Source: CAD feature listing. Evaluate the final solid. Frame: model axes, mm. A direction names the side the tool comes from. Give positions to 0.01 mm unless a question says otherwise; leave off trailing zeros. Write each loop counter-clockwise with the first axis right and the second up, starting at its lowest first coordinate (ties: lowest second). Pieces come first, ordered by that corner, then holes. Notation, with made-up numbers: (19.25, 14) -> (55.25, 14) arc R31 cw to (55.25, 46) -> close; hole circle Ø1 at (76.25, 79.5). An arc over 180 degrees is marked (long way). Answer as a JSON object with one key per item and string values. Group by question number.
Item 1: First-contact query: pin 1 Ø5 at (x, z) = (40.5, -44.5) entering from +Y; pin 2 Ø1.7 at (y, z) = (15, -40.9) entering from +X; pin 3 Ø4 at (y, z) = (14, -47) entering from -X; pin 4 Ø4 at (x, y) = (29.5, 23) entering from -Z. Flat tips, straight axial feed; report the tip coordinate or a pass-through.
Item 2: Access query for faces 4 (the face through (43.5, 17.7, -54.8)), 5 (the face through (45.2, 15, -41)), 6 (the face through (32, 15, -6)), 7 (the face through (19.8, 22, -43)). Directions: +Z, -Z, +X, -X, +Y, -Y. A direction counts if a zero-diameter tool reaches every point of the face in a straight line with its end or side. Return the directions, or none.
Item 3: Section query A-A on z = -48.34. Return the cut outline in (x, y), plus the area to 3 significant figures.
Item 4: Section query B-B on y = 15. Return the cut outline in (x, z), plus the area to 3 significant figures.
Item 5: Section query D-D on y = 5.5. Return the cut outline in (x, z), plus the area to 4 significant figures.
Item 6: Section query C-C on z = -30. Return the cut outline in (x, y), plus the area to 3 significant figures.
Item 7: Ray query, probe 1 along X at (y, z) = (25, -13); probe 2 along Y at (x, z) = (43.25, -48.34); probe 3 along Y at (x, z) = (47.75, -40.9). Return the intervals inside material, ascending. Write a range as from..to.
Item 8: Pull-direction query (Z, two-part tool) for faces 1 (the face through (31, 15, -11)), 2 (the face through (41.6, 22, -43)), 3 (the face through (47.228, 15.279, -56.667)); classes: pulls with the +Z half, pulls with the -Z half, needs draft (parallel to the pull), parting line crosses it, or undercut.
from build123d import *

# Parameters (mm, degrees)
SKETCH1_W           = 5
SKETCH1_H           = 70
SKETCH1_W_2         = 40
SKETCH1_H_2         = 5
BOSS_EXTRUDE1_DEPTH = 30
SKETCH2_R           = 7
CUT_EXTRUDE1_DEPTH  = 70
SKETCH3_W           = 111.167782235
SKETCH3_H           = 40.74685258
CUT_EXTRUDE2_DEPTH  = 0.8
SKETCH5_W           = 117.774687649
SKETCH5_H           = 158.291815666
CUT_EXTRUDE3_DEPTH  = 0.8
SKETCH6_W           = 70
SKETCH6_H           = 30
BOSS_EXTRUDE2_DEPTH = 3.4
SKETCH7_W           = 70
SKETCH7_H           = 30
BOSS_EXTRUDE3_DEPTH = 6.7
SKETCH8_W           = 83.763231722
SKETCH8_H           = 77.916949986
CUT_EXTRUDE5_DEPTH  = 6
SKETCH9_R           = 7
CUT_EXTRUDE6_DEPTH  = 90.354574589
SKETCH10_W          = 29.9
SKETCH10_H          = 30
BOSS_EXTRUDE4_DEPTH = 6
SKETCH11_W          = 55.967068903
SKETCH11_H          = 62.229878259
CUT_EXTRUDE7_DEPTH  = 6
SKETCH12_W          = 64
SKETCH12_H          = 30
BOSS_EXTRUDE6_DEPTH = 4.05
SKETCH13_W          = 85.617860434
SKETCH13_H          = 123.38327663
CUT_EXTRUDE9_DEPTH  = 4.05
SKETCH15_W          = 39.049263631
SKETCH15_H          = 151.632152685
CUT_EXTRUDE10_DEPTH = 3.95
SKETCH16_W          = 64
SKETCH16_H          = 30
BOSS_EXTRUDE7_DEPTH = 4.05
SKETCH17_W          = 96.474130843
SKETCH17_H          = 104.566259817
CUT_EXTRUDE11_DEPTH = 4.05
SKETCH18_W          = 6.755230809
SKETCH18_H          = 55.059186595
CUT_EXTRUDE12_DEPTH = 4.05
SKETCH19_R          = 7
CUT_EXTRUDE14_DEPTH = 34.05
SKETCH23_W          = 19.849593964
SKETCH23_H          = 19.85515092
BOSS_EXTRUDE9_DEPTH = 4.2
SKETCH24_R          = 0.93
CUT_EXTRUDE16_DEPTH = 4
SKETCH24_5_R        = 0.93
CUT_EXTRUDE17_DEPTH = 4
SKETCH26_R          = 7
CUT_EXTRUDE18_DEPTH = 0.4


with BuildPart() as part:
    # Sketch1 → Boss-Extrude1 (new body)
    with BuildSketch(Plane(origin=(0, 0, 0), x_dir=(1, 0, 0), z_dir=(0, 1, 0))):
        with Locations((2.5, 40)):
            Rectangle(SKETCH1_W, SKETCH1_H)
        with Locations((25, 2.5)):
            Rectangle(SKETCH1_W_2, SKETCH1_H_2)
        with Locations((2.5, 2.5)):
            Rectangle(SKETCH1_W, SKETCH1_H_2)
        with Locations((47.5, 40)):
            Rectangle(SKETCH1_W, SKETCH1_H)
        with Locations((47.5, 2.5)):
            Rectangle(SKETCH1_W, SKETCH1_H_2)
    extrude(amount=BOSS_EXTRUDE1_DEPTH)

    # Sketch2 → Cut-Extrude1 (cut)
    with BuildSketch(Plane(origin=(50, 0, 0), x_dir=(0, 0, -1), z_dir=(1, 0, 0))):
        with Locations(Location((48.34, 15, 0), (0, 0, 180))):
            Circle(SKETCH2_R)
    extrude(amount=-CUT_EXTRUDE1_DEPTH, mode=Mode.SUBTRACT)

    # Sketch3 → Cut-Extrude2 (cut)
    with BuildSketch(Plane(origin=(50, 0, 0), x_dir=(0, 0, -1), z_dir=(1, 0, 0))):
        with Locations((37.634857553, 15.397923555)):
            Rectangle(SKETCH3_W, SKETCH3_H)
    extrude(amount=-CUT_EXTRUDE2_DEPTH, mode=Mode.SUBTRACT)

    # Sketch5 → Cut-Extrude3 (cut)
    with BuildSketch(Plane.ZY):
        with Locations((-53.14418593, -0.770080807)):
            Rectangle(SKETCH5_W, SKETCH5_H)
    extrude(amount=-CUT_EXTRUDE3_DEPTH, mode=Mode.SUBTRACT)

    # Sketch6 → Boss-Extrude2 (add)
    with BuildSketch(Plane.ZY.offset(-45)):
        with Locations((-40, 15)):
            Rectangle(SKETCH6_W, SKETCH6_H)
    extrude(amount=BOSS_EXTRUDE2_DEPTH)

    # Sketch7 → Boss-Extrude3 (add)
    with BuildSketch(Plane(origin=(5, 0, 0), x_dir=(0, 0, -1), z_dir=(1, 0, 0))):
        with Locations((40, 15)):
            Rectangle(SKETCH7_W, SKETCH7_H)
    extrude(amount=BOSS_EXTRUDE3_DEPTH)

    # Sketch8 → Cut-Extrude5 (cut)
    with BuildSketch(Plane.ZY.offset(-0.8)):
        with Locations((-33.178908474, 22.347774268)):
            Rectangle(SKETCH8_W, SKETCH8_H)
    extrude(amount=-CUT_EXTRUDE5_DEPTH, mode=Mode.SUBTRACT)

    # Sketch9 → Cut-Extrude6 (cut, through all)
    with BuildSketch(Plane(origin=(45, 0, 0), x_dir=(0, 0, -1), z_dir=(1, 0, 0))):
        with Locations((48.34, 15)):
            Circle(SKETCH9_R)
    extrude(amount=-CUT_EXTRUDE6_DEPTH, mode=Mode.SUBTRACT)

    # Sketch10 → Boss-Extrude4 (add)
    with BuildSketch(Plane(origin=(0, 0, -5), x_dir=(-1, 0, 0), z_dir=(0, 0, -1))):
        with Locations((-26.65, 15)):
            Rectangle(SKETCH10_W, SKETCH10_H)
    extrude(amount=BOSS_EXTRUDE4_DEPTH)

    # Sketch11 → Cut-Extrude7 (cut)
    with BuildSketch(Plane.XY):
        with Locations((27.983534452, 15.70224338)):
            Rectangle(SKETCH11_W, SKETCH11_H)
    extrude(amount=-CUT_EXTRUDE7_DEPTH, mode=Mode.SUBTRACT)

    # Sketch12 → Boss-Extrude6 (add)
    with BuildSketch(Plane(origin=(11.7, 0, 0), x_dir=(0, 0, -1), z_dir=(1, 0, 0))):
        with Locations((43, 15)):
            Rectangle(SKETCH12_W, SKETCH12_H)
    extrude(amount=BOSS_EXTRUDE6_DEPTH)

    # Sketch13 → Cut-Extrude9 (cut)
    with BuildSketch(Plane.ZY.offset(-6.8)):
        with Locations((-48.94815067, 16.542324461)):
            Rectangle(SKETCH13_W, SKETCH13_H)
    extrude(amount=-CUT_EXTRUDE9_DEPTH, mode=Mode.SUBTRACT)

    # Sketch15 → Cut-Extrude10 (cut)
    with BuildSketch(Plane.ZY.offset(-6.8)):
        with Locations((0.466031991, 2.740241295)):
            Rectangle(SKETCH15_W, SKETCH15_H)
    extrude(amount=-CUT_EXTRUDE10_DEPTH, mode=Mode.SUBTRACT)

    # Sketch16 → Boss-Extrude7 (add)
    with BuildSketch(Plane(origin=(15.75, 0, 0), x_dir=(0, 0, -1), z_dir=(1, 0, 0))):
        with Locations((43, 15)):
            Rectangle(SKETCH16_W, SKETCH16_H)
    extrude(amount=BOSS_EXTRUDE7_DEPTH)

    # Sketch17 → Cut-Extrude11 (cut)
    with BuildSketch(Plane.ZY.offset(-10.85)):
        with Locations((-42.673680758, 11.569509922)):
            Rectangle(SKETCH17_W, SKETCH17_H)
    extrude(amount=-CUT_EXTRUDE11_DEPTH, mode=Mode.SUBTRACT)


with BuildPart() as cut_extrude11_piece_1:
    # of the separate pieces the step leaves, piece 1, a body of its own (cut_extrude11_pieces)
    add(part.part.solids().sort_by_distance((19.8, 0, -75))[0])

    # Sketch19 → Cut-Extrude14 (cut)
    with BuildSketch(Plane(origin=(19.8, 0, 0), x_dir=(0, 0, -1), z_dir=(1, 0, 0))):
        with Locations((48.34, 15)):
            Circle(SKETCH19_R)
    extrude(amount=-CUT_EXTRUDE14_DEPTH, mode=Mode.SUBTRACT)

    # Sketch23 → Boss-Extrude9 (add)
    with BuildSketch(Plane(origin=(49.2, 0, 0), x_dir=(0, 0, -1), z_dir=(1, 0, 0))):
        with Locations((46.616592264, 15.948021262)):
            Rectangle(SKETCH23_W, SKETCH23_H)
    extrude(amount=-BOSS_EXTRUDE9_DEPTH)

    # Sketch24 → Cut-Extrude16 (cut)
    with BuildSketch(Plane(origin=(49.2, 0, 0), x_dir=(0, 0, -1), z_dir=(1, 0, 0))):
        with Locations((55.78, 15)):
            Circle(SKETCH24_R)
    extrude(amount=-CUT_EXTRUDE16_DEPTH, mode=Mode.SUBTRACT)

    # Sketch24_5 → Cut-Extrude17 (cut)
    with BuildSketch(Plane(origin=(49.2, 0, 0), x_dir=(0, 0, -1), z_dir=(1, 0, 0))):
        with Locations((40.9, 15)):
            Circle(SKETCH24_5_R)
    extrude(amount=-CUT_EXTRUDE17_DEPTH, mode=Mode.SUBTRACT)

    # Sketch26 → Cut-Extrude18 (cut)
    with BuildSketch(Plane.ZY.offset(-45)):
        with Locations(Location((-48.34, 15, 0), (0, 0, 180))):
            Circle(SKETCH26_R)
    extrude(amount=-CUT_EXTRUDE18_DEPTH, mode=Mode.SUBTRACT)


with BuildPart() as cut_extrude11_piece_2:
    # of the separate pieces the step leaves, piece 2, a body of its own (cut_extrude11_pieces)
    add(part.part.solids().sort_by_distance((10.85, 0, -6))[0])

    # Sketch18 → Cut-Extrude12 (cut)
    with BuildSketch(Plane.ZY.offset(-10.75)):
        with Locations((-5.990573003, 11.129995274)):
            Rectangle(SKETCH18_W, SKETCH18_H)
    extrude(amount=-CUT_EXTRUDE12_DEPTH, mode=Mode.SUBTRACT)


solid = cut_extrude11_piece_1.part
Worked answers:
{
 "1": {"pin 1": "y = 30", "pin 2": "x = 45.2", "pin 3": "x = 45.4", "pin 4": "z = -11"},
 "2": {"face 4": "-X", "face 5": "+X", "face 6": "+Z, +X, -X, +Y, -Y", "face 7": "-Z, +Y, -Y"},
 "3": {"outline": "(14.9, 0) -> (19.8, 0) -> (19.8, 8) -> (14.9, 8) -> close; (14.9, 22) -> (19.8, 22) -> (19.8, 30) -> (14.9, 30) -> close; (41.6, 0) -> (49.2, 0) -> (49.2, 30) -> (41.6, 30) -> (41.6, 22) -> (45.4, 22) -> (45.4, 8) -> (41.6, 8) -> close", "area": "253 mm^2"},
 "4": {"outline": "(14.9, -75) -> (19.8, -75) -> (19.8, -55.34) -> (14.9, -55.34) -> close; (14.9, -41.34) -> (19.8, -41.34) -> (19.8, -11) -> (41.6, -11) -> (41.6, -41.34) -> (45.2, -41.34) -> (45.2, -39.97) -> (49.2, -39.97) -> (49.2, -6) -> (14.9, -6) -> close; (41.6, -75) -> (49.2, -75) -> (49.2, -56.71) -> (45.2, -56.71) -> (45.2, -55.34) -> (41.6, -55.34) -> close; (45.4, -54.85) -> (49.2, -54.85) -> (49.2, -41.83) -> (45.4, -41.83) -> close", "area": "835 mm^2"},
 "5": {"outline": "(14.9, -75) -> (19.8, -75) -> (19.8, -11) -> (41.6, -11) -> (41.6, -75) -> (49.2, -75) -> (49.2, -6) -> (14.9, -6) -> close", "area": "971.5 mm^2"},
 "6": {"outline": "(14.9, 0) -> (19.8, 0) -> (19.8, 30) -> (14.9, 30) -> close; (41.6, 0) -> (49.2, 0) -> (49.2, 30) -> (41.6, 30) -> close", "area": "375 mm^2"},
 "7": {"probe 1": "14.9..19.8, 41.6..49.2", "probe 2": "0..8, 22..30", "probe 3": "0..14.07, 15.93..30"},
 "8": {"face 1": "pulls with the -Z half", "face 2": "needs draft", "face 3": "undercut"}
}
